The drawing under review shows one solid part. Ordinate dimensions are in mm from its lowest x, y, z. Give positions to 0.01 mm unless a question says otherwise; leave off trailing zeros. Order: outer loops, then holes, each group sorted by start corner. A loop starts at its lowest first (then second) coordinate and runs counter-clockwise, first axis right, second up. Notation, with made-up numbers: (-32, -37) -> (19, -37) arc R14 cw to (19, -20) -> close; hole circle Ø5 at (46.25, 26.5). An arc over 180 degrees is marked (long way). Use CSV: the item, a comma, the result in double quotes. Start each with the question number.
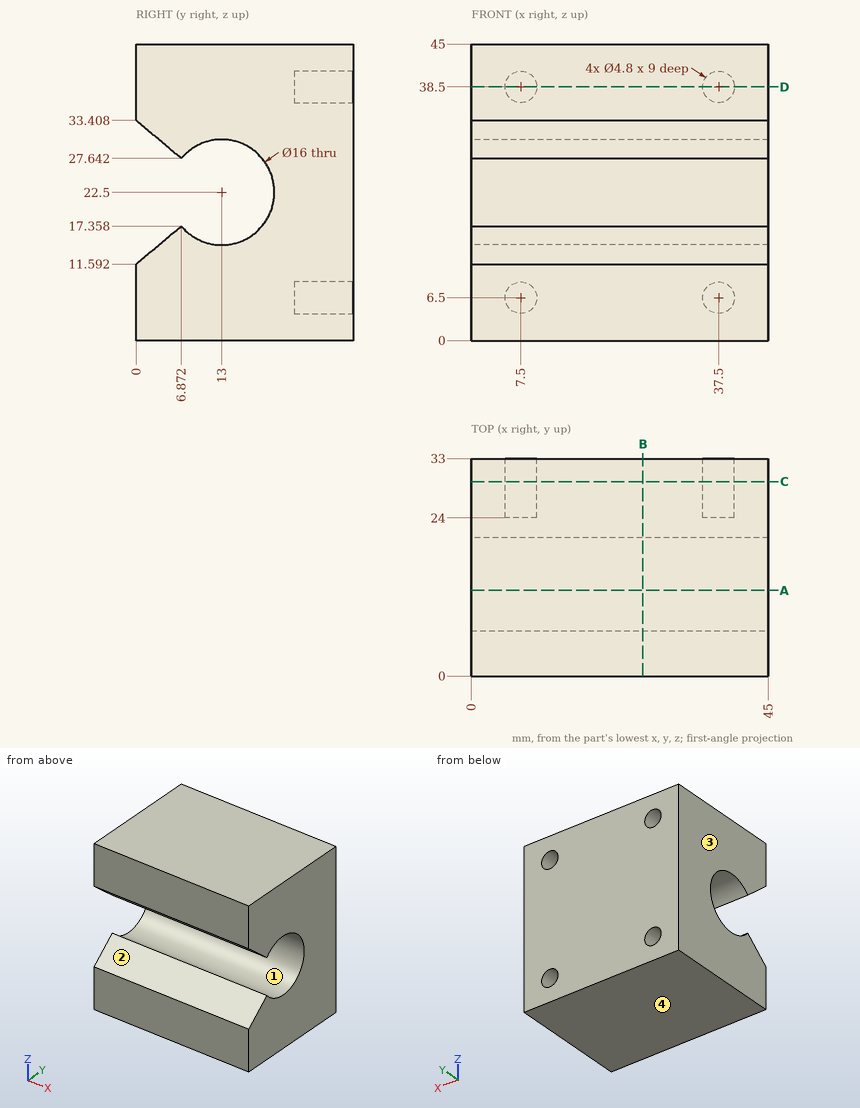
1. Clearance check with flat-ended pins moving along their axes: P1, Ø12, axis at x = 7, y = 5.5, coming from the -Z side; P2, Ø1.4, axis at x = 38.5, z = 6.5, coming from the +Y side. State where each tip first meets the part, or that it passes through.
2. Consider section B-B (x = 26). State the section outline as (y, z) points.
3. Consider section A-A (y = 13). State the section outline as (x, z) points.
4. Consider section C-C (y = 29.5). State the section outline as (x, z) points, plus the area to 3 significant figures.
5. Draft analysis for pull direction Z (two halves, no side actions). For the marked faces 1, 2, 3 and 4, state which applies: +Z half, -Z half, draft (parallel to the pull), parting line (faces both ways), or undercut.
6. Consider section D-D (z = 38.5). State the section outline as (x, y) points, plus the area to 3 significant figures.
7. To check wall thickness, follow L1, parallel to X at y = 29.5, z = 38.5; L2, parallel to Z at x = 3.5, y = 13; L3, parallel to X at y = 32.5, z = 40.5 (1 decimal). State the ranges of each line that lie inside material, in increasing order. Write a range as [from, to].
Answer list:
1,P1,"z = 0"
1,P2,"y = 24"
2,outline,"(0, 0) -> (33, 0) -> (33, 45) -> (0, 45) -> (0, 33.41) -> (6.87, 27.64) arc R8 cw (long way) to (6.87, 17.36) -> (0, 11.59) -> close"
3,outline,"(0, 0) -> (45, 0) -> (45, 14.5) -> (0, 14.5) -> close; (0, 30.5) -> (45, 30.5) -> (45, 45) -> (0, 45) -> close"
4,outline,"(0, 0) -> (45, 0) -> (45, 45) -> (0, 45) -> close; hole circle Ø4.8 at (7.5, 6.5); hole circle Ø4.8 at (7.5, 38.5); hole circle Ø4.8 at (37.5, 6.5); hole circle Ø4.8 at (37.5, 38.5)"
4,area,"1,950 mm2"
5,face 1,"undercut"
5,face 2,"undercut"
5,face 3,"draft"
5,face 4,"-Z half"
6,outline,"(0, 0) -> (45, 0) -> (45, 33) -> (39.9, 33) -> (39.9, 24) -> (35.1, 24) -> (35.1, 33) -> (9.9, 33) -> (9.9, 24) -> (5.1, 24) -> (5.1, 33) -> (0, 33) -> close"
6,area,"1,400 mm2"
7,L1,"[0, 5.1], [9.9, 35.1], [39.9, 45]"
7,L2,"[0, 14.5], [30.5, 45]"
7,L3,"[0, 6.2], [8.8, 36.2], [38.8, 45]"
